The model under review builds one solid part; all positions refer to its coordinate system, in mm. A direction names the side the tool comes from. Coordinates: 2 decimals unless noted, no trailing zeros. Order: outer loops, then holes, each group sorted by start corner. A loop starts at its lowest first (then second) coordinate and runs counter-clockwise, first axis right, second up. Notation, with made-up numbers: (-1.75, -22.75) - (42.25, -22.75) arc R24 ccw to (42.25, 5.25) - close; hole circle Ø8 at (11.5, 12.25). An arc over 180 degrees is marked (long way). Answer in a Markdown table with one row per item.
```python
from build123d import *

# Parameters (mm, degrees)
SKETCH2_R          = 2.5
CUT_EXTRUDE1_DEPTH = 4.5
SKETCH4_R          = 8.5
CUT_EXTRUDE3_DEPTH = 2


with BuildPart() as part:
    # Sketch1 → Revolve1 (revolve)
    with BuildSketch(Plane.XY, mode=Mode.PRIVATE) as revolve1_sk:
        Polygon((0, 30), (6, 30), (6, 24.55), (7, 24.55), (7, 20.55), (18, 20.55), (18, 6.5), (6, 6.5), (6, 7.5), (0, 7.5), align=None)
    revolve(revolve1_sk.sketch.rotate(Axis((0, 0, 0), (1, 0, 0)), 90), axis=Axis((0, 0, 0), (1, 0, 0)))

    # Sketch2 → Cut-Extrude1 (cut)
    with BuildSketch(Plane.ZY):
        with Locations((0, 20)):
            Circle(SKETCH2_R)
        with Locations((17.320508076, 10)):
            Circle(SKETCH2_R)
        with Locations((17.320508076, -10)):
            Circle(SKETCH2_R)
        with Locations((0, -20)):
            Circle(SKETCH2_R)
        with Locations((-17.320508076, -10)):
            Circle(SKETCH2_R)
        with Locations((-17.320508076, 10)):
            Circle(SKETCH2_R)
    extrude(amount=-CUT_EXTRUDE1_DEPTH, mode=Mode.SUBTRACT)

    # Sketch4 → Cut-Extrude3 (cut)
    with BuildSketch(Plane.ZY):
        Circle(SKETCH4_R)
    extrude(amount=-CUT_EXTRUDE3_DEPTH, mode=Mode.SUBTRACT)


solid = part.part
```
Item 1: We need section C-C, the plane x = 14.5. Write out the cut boundary in (y, z).
Check values:
| item | result |
|---|---|
| outline | circle Ø41.1 at (0, 0); hole circle Ø13 at (0, 0) |
Item 2: To check wall thickness, follow line 1 (Y direction, x = 13.5, z = 0); line 2 (X direction, y = 12.5, z = -20.5); line 3 (X direction, y = 23, z = 13.5). State the ranges of each line that lie inside material, in increasing order. Write a range as from..to.
Check values:
| item | result |
|---|---|
| line 1 | -20.55..-6.5, 6.5..20.55 |
| line 2 | 0..7 |
| line 3 | 0..6 |
Item 3: Clearance check with flat-ended pins moving along their axes: pin 1 Ø4 at (y, z) = (-21, -0.5) entering from -X; pin 2 Ø2.5 at (y, z) = (19, 0.5) entering from -X; pin 3 Ø7.5 at (y, z) = (-1.5, 3) entering from -X; pin 4 Ø10 at (x, y) = (13.5, -18.5) entering from +Z. State where each tip first meets the part, or that it passes through.
Check values:
| item | result |
|---|---|
| pin 1 | x = 0 |
| pin 2 | x = 4.5 |
| pin 3 | x = 6 |
| pin 4 | z = 15.49 |
Item 4: We need section D-D, the plane z = -18. Write out the cut boundary in (x, y), then the cut area to 3 significant figures.
Check values:
| item | result |
|---|---|
| outline | (0, -24) - (6, -24) - (6, -16.69) - (7, -16.69) - (7, -9.91) - (18, -9.91) - (18, 9.91) - (7, 9.91) - (7, 16.69) - (6, 16.69) - (6, 24) - (0, 24) - (0, 12.41) - (4.5, 12.41) - (4.5, 7.59) - (0, 7.59) - (0, -7.59) - (4.5, -7.59) - (4.5, -12.41) - (0, -12.41) - close |
| area | 496 mm^2 |
Item 5: Mouldability with a two-part tool opening along Y and no side actions: class faces 3 (the face through (6.51, 21.78, 11.33)), 4 (the face through (11.916, 3.955, -5.158)), 5 (the face through (2.218, 9.042, -15.011)), 6 (the face through (6, 0, -25)) as +Y half, -Y half, draft (parallel to the pull), parting line (faces both ways), or undercut.
Check values:
| item | result |
|---|---|
| face 3 | parting line |
| face 4 | undercut |
| face 5 | undercut |
| face 6 | draft |
Item 6: Tool access review of faces 1 (the face through (3.042, -25.296, 16.128)), 2 (the face through (4.5, 10, -17)): name each direction out of +Z, -Z, +X, -X, +Y, -Y from which nothing blocks a thin tool from reaching the whole face with its end or side.
Check values:
| item | result |
|---|---|
| face 1 | +X, -X |
| face 2 | -X |
Item 7: We need section A-A, the plane y = 0. Write out the cut boundary in (x, z).
Check values:
| item | result |
|---|---|
| outline | (0, -30) - (6, -30) - (6, -24.55) - (7, -24.55) - (7, -20.55) - (18, -20.55) - (18, -6.5) - (6, -6.5) - (6, -7.5) - (2, -7.5) - (2, -8.5) - (0, -8.5) - close; (0, 8.5) - (2, 8.5) - (2, 7.5) - (6, 7.5) - (6, 6.5) - (18, 6.5) - (18, 20.55) - (7, 20.55) - (7, 24.55) - (6, 24.55) - (6, 30) - (0, 30) - close |
